Part print with two shaded views. Sizes in mm from the minimum x, y, z corner. A direction names the side the tool comes from. Coordinates: 2 decimals unless noted, no trailing zeros. Loops run counter-clockwise (first coordinate to the right, second up) from the corner with the lowest first, then second, coordinate; pieces in that order, holes last. Notation, with made-up numbers: (71, 88) -> (113, 88) arc R20 cw to (113, 125) -> close; hole circle Ø9 at (-9, 68.25). An arc over 180 degrees is marked (long way). Return JSON: item names as keys, results as strings. Group by question number.
(1) Tool access for the marked faces 4 and 5: list every direction of +Z, -Z, +X, -X, +Y, -Y with a clear straight run to the whole face (end or side of a thin tool).
(2) Saw through at D-D on z = 19.5. Write the cut outline in (x, y).
(3) Saw through at A-A on x = 15. Write the cut outline in (y, z).
(4) Probe L1, parallel to Y at x = 15, z = 13.25; L2, parallel to Z at x = 13, y = 10.5; L3, parallel to X at y = 21.5, z = 8.25. List the from-to ranges inside material, lowest first.
(5) Mould opens along Y. For the marked faces 1, 2 and 3 say: pulls with the +Y half, pulls with the -Y half, needs draft (parallel to the pull), parting line crosses it, or undercut.
(6) Flat gauge pins, fed straight in: pin 1 Ø10 at (y, z) = (19.5, 17) entering from -X; pin 2 Ø5 at (x, z) = (20, 17) entering from +Y; pin 3 Ø2 at (y, z) = (15, 16.5) entering from +X. Where does each tip first touch, or does it go through?
(7) Saw through at C-C on z = 4. Write the cut outline in (x, y).
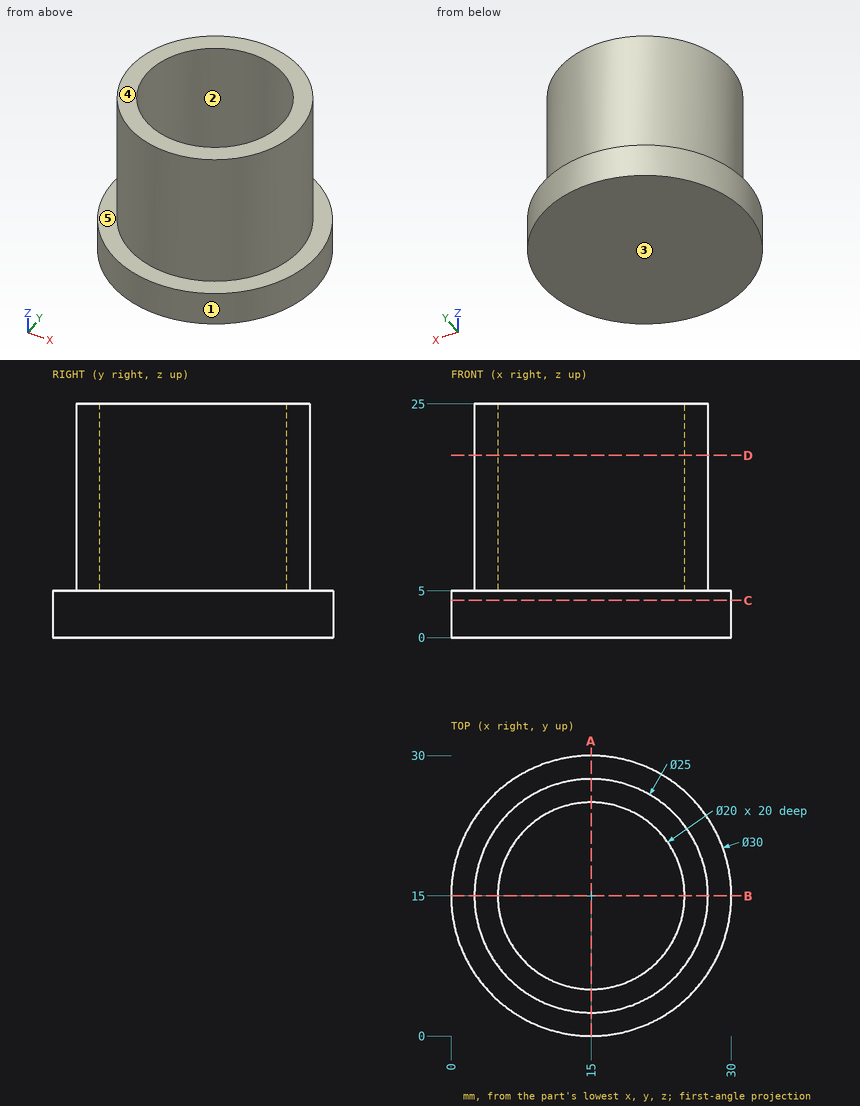
Geometry results:
{
 "1": {"face 4": "+Z, +X, -X, +Y, -Y", "face 5": "+Z"},
 "2": {"outline": "circle Ø25 at (15, 15); hole circle Ø20 at (15, 15)"},
 "3": {"outline": "(0, 0) -> (30, 0) -> (30, 5) -> (27.5, 5) -> (27.5, 25) -> (25, 25) -> (25, 5) -> (5, 5) -> (5, 25) -> (2.5, 25) -> (2.5, 5) -> (0, 5) -> close"},
 "4": {"L1": "2.5 to 5, 25 to 27.5", "L2": "0 to 5", "L3": "4.32 to 7.4, 22.6 to 25.68"},
 "5": {"face 1": "parting line crosses it", "face 2": "undercut", "face 3": "needs draft"},
 "6": {"pin 1": "x = 2.5", "pin 2": "y = 27.25", "pin 3": "x = 27.5"},
 "7": {"outline": "circle Ø30 at (15, 15)"}
}
